Model file for the job. Use its own axes, mm. A direction names the side the tool comes from. Give positions to 0.01 mm unless a question says otherwise; leave off trailing zeros. Order: outer loops, then holes, each group sorted by start corner. A loop starts at its lowest first (then second) coordinate and runs counter-clockwise, first axis right, second up. Notation, with made-up numbers: (-37, 21) - (-23, 21) arc R16 ccw to (-23, 33) - close; hole circle Ø10 at (-28, 45). An arc over 180 degrees is marked (long way). Use CSV: the item, a comma, the result in double quotes. Start each with the question number.
(1) Probe L1, parallel to Y at x = 48.5, z = -9.25; L2, parallel to Z at x = -5, y = 6; L3, parallel to Y at x = 2.5, z = 7.25. List the from-to ranges inside material, lowest first.
(2) Tool access for faces 1 (the flat face through (44, 13, 4)), 2 (the flat face through (0, 13, 4)), 3 (the flat face through (22, 0, 4)): list every direction of +Z, -Z, +X, -X, +Y, -Y with a clear straight run to the whole face (end or side of a thin tool).
(3) Band-saw the part on D-D, the plane z = 5. Give the cut face in (x, y).
(4) Band-saw the part on A-A, the plane x = -4.5. Give the cut face in (y, z), then the cut area to 3 significant figures.
(5) Pull direction Y, two halves, no side cores. Call faces 4 (the flat face through (22, 26, 4)), 5 (the cylindrical face through (-5.886, -0.575, -7.395)), 6 (the flat face through (22, -2, 0)), 7 (the cylindrical face through (49.61, 27.01, -7.4)): +Y half, -Y half, draft (parallel to the pull), parting line (faces both ways), or undercut.
(6) Band-saw the part on C-C, the plane x = 8. Give the cut face in (y, z).
(7) Band-saw the part on B-B, the plane y = 13. Give the cut face in (x, z).
(8) Drop flat-ended pins along their axis: pin 1 Ø2.5 at (y, z) = (17, 3) entering from -X; pin 2 Ø10 at (x, z) = (21, 6.5) entering from -Y; pin 3 Ø2.5 at (x, z) = (12.5, 6) entering from +Y. Give the stop position or say it passes through.
from build123d import *

# Parameters (mm, degrees)
CROQUIS1_W              = 44
CROQUIS1_H              = 26
SALIENTE_EXTRUIR1_DEPTH = 9
CROQUIS2_W              = 60
CROQUIS2_H              = 35
CROQUIS2_R              = 1.5
SALIENTE_EXTRUIR2_DEPTH = 15


with BuildPart() as part:
    # Croquis1 → Saliente-Extruir1 (new body)
    with BuildSketch(Plane.XY):
        with Locations((22, 13)):
            Rectangle(CROQUIS1_W, CROQUIS1_H)
    extrude(amount=SALIENTE_EXTRUIR1_DEPTH)

    # Croquis2 → Saliente-Extruir2 (add)
    with BuildSketch(Plane(origin=(0, 0, 0), x_dir=(-1, 0, 0), z_dir=(0, 0, -1))):
        with Locations((-22, 13)):
            Rectangle(CROQUIS2_W, CROQUIS2_H)
        with Locations((-48.5, 26)):
            Circle(CROQUIS2_R, mode=Mode.SUBTRACT)
        with Locations((4.5, 26)):
            Circle(CROQUIS2_R, mode=Mode.SUBTRACT)
        with Locations((-48.5, 0)):
            Circle(CROQUIS2_R, mode=Mode.SUBTRACT)
        with Locations((4.5, 0)):
            Circle(CROQUIS2_R, mode=Mode.SUBTRACT)
    extrude(amount=SALIENTE_EXTRUIR2_DEPTH)


solid = part.part
Answer block:
1,L1,"y = -4.5 to -1.5, 1.5 to 24.5, 27.5 to 30.5"
1,L2,"z = -15 to 0"
1,L3,"y = 0 to 26"
2,face 1,"+Z, +X, +Y, -Y"
2,face 2,"+Z, -X, +Y, -Y"
2,face 3,"+Z, +X, -X, -Y"
3,outline,"(0, 0) - (44, 0) - (44, 26) - (0, 26) - close"
4,outline,"(-4.5, -15) - (-1.5, -15) - (-1.5, 0) - (-4.5, 0) - close; (1.5, -15) - (24.5, -15) - (24.5, 0) - (1.5, 0) - close; (27.5, -15) - (30.5, -15) - (30.5, 0) - (27.5, 0) - close"
4,area,"435 mm2"
5,face 4,"+Y half"
5,face 5,"undercut"
5,face 6,"draft"
5,face 7,"undercut"
6,outline,"(-4.5, -15) - (30.5, -15) - (30.5, 0) - (26, 0) - (26, 9) - (0, 9) - (0, 0) - (-4.5, 0) - close"
7,outline,"(-8, -15) - (52, -15) - (52, 0) - (44, 0) - (44, 9) - (0, 9) - (0, 0) - (-8, 0) - close"
8,pin 1,"stops at x = 0"
8,pin 2,"stops at y = 0"
8,pin 3,"stops at y = 26"
